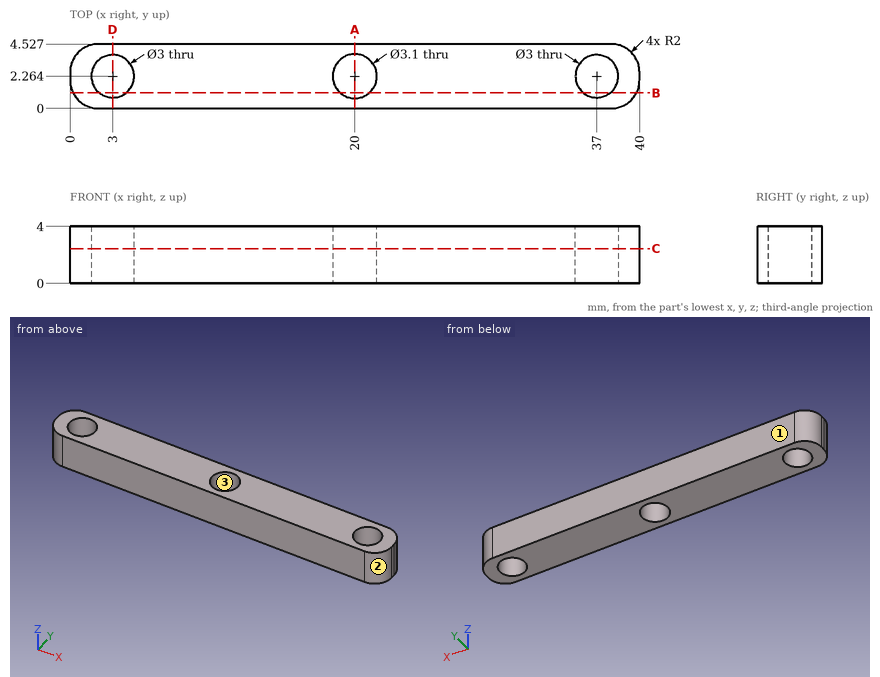
Could you check a few things on this drawing? It's one solid part, dimensions in mm from its lowest x, y, z. Coordinates: 2 decimals unless noted, no trailing zeros. Order: outer loops, then holes, each group sorted by start corner. A loop starts at its lowest first (then second) coordinate and runs counter-clockwise, first axis right, second up. Notation, with made-up numbers: M 58,47.25 L 68,47.25 A17 ccw 68,58.25 Z; hole C 46.25,58.5 d6. An arc over 180 degrees is marked long. Answer as a JSON object with one key per item and string values. Group by question number.
(1) If we mould it in two halves opening along X, with no side actions, what happens to the marked faces 1, 2 and 3? For each: released by +X, released by -X, zero draft, split by the parting line, or undercut.
(2) Suppose I cut it at B-B, the plane y = 1.1. Please give me the cut outline in (x, z), then the cut area to 3 significant figures.
(3) Suppose I cut it at D-D, the plane x = 3. Please give me the cut outline in (y, z).
(4) Suppose I cut it at C-C, the plane z = 2.45. Please give me the cut outline in (x, y).
(5) Suppose I cut it at A-A, the plane x = 20. Please give me the cut outline in (y, z).
(6) I need wall thicknesses on probe 1 along Y at (x, z) = (20, 1.95); probe 2 along Y at (x, z) = (3, 2.8); probe 3 along X at (y, z) = (1.6, 2) (1 decimal). Which ranges of each line are inside material? Lowest first, please.
Values found:
{
 "1": {"face 1": "zero draft", "face 2": "released by +X", "face 3": "undercut"},
 "2": {"outline": "M 0.21,0 L 2.05,0 L 2.05,4 L 0.21,4 Z; M 3.95,0 L 18.98,0 L 18.98,4 L 3.95,4 Z; M 21.02,0 L 36.05,0 L 36.05,4 L 21.02,4 Z; M 37.95,0 L 39.79,0 L 39.79,4 L 37.95,4 Z", "area": "135 mm^2"},
 "3": {"outline": "M 0,0 L 0.76,0 L 0.76,4 L 0,4 Z; M 3.76,0 L 4.53,0 L 4.53,4 L 3.76,4 Z"},
 "4": {"outline": "M 0,2 A2 ccw 2,0 L 38,0 A2 ccw 40,2 L 40,2.53 A2 ccw 38,4.53 L 2,4.53 A2 ccw 0,2.53 Z; hole C 3,2.26 d3; hole C 20,2.26 d3.1; hole C 37,2.26 d3"},
 "5": {"outline": "M 0,0 L 0.71,0 L 0.71,4 L 0,4 Z; M 3.81,0 L 4.53,0 L 4.53,4 L 3.81,4 Z"},
 "6": {"probe 1": "y = 0 to 0.71, 3.81 to 4.53", "probe 2": "y = 0 to 0.76, 3.76 to 4.53", "probe 3": "x = 0 to 1.7, 4.3 to 18.6, 21.4 to 35.7, 38.3 to 40"}
}
